Part model, mm, in its own coordinate system. A direction names the side the tool comes from. Round coordinates to 2 decimals unless told otherwise and drop trailing zeros. Write each loop counter-clockwise with the first axis right and the second up, starting at its lowest first coordinate (ties: lowest second). Pieces come first, ordered by that corner, then holes. Notation, with made-up numbers: M 37.5,69.5 L 81.5,69.5 A25 cw 81.5,91.5 Z; hole C 27.25,26 d8. An arc over 180 degrees is marked long. Use a Markdown table: item, result. Add a question column.
1) Which spindle directions (+Z, -Z, +X, -X, +Y, -Y) get a long thin tool onto all of the face, cutting with end or side? Do faces 5 (the face through (10, 31.1, -15)), 6 (the face through (22.1, 4.5, -13)), 7 (the face through (7.535, 129.651, -14.58)). Say none if no direction does.
2) Slice it at D-D on z = -15. Give the number of separate pieces and of enclosed holes in the cut face, plus the area to 3 significant figures.
3) Wall check: probe 1 along Y at (x, z) = (25, -15) (3 decimals); probe 2 along Y at (x, z) = (21.45, -15) (1 decimal); probe 3 along Z at (x, y) = (24, 23.56). Give the ranges that are in metal, low to high.
4) Two-plate mould, pull along Z, no slides. Class faces 1 (the face through (22.1, 21.5, -13)), 2 (the face through (15, 28, -30)), 3 (the face through (5.39, 116.48, -14.58)), 4 (the face through (15, 28, 0)): released by +Z, released by -Z, zero draft, split by the parting line, or undercut.
5) Slice it at A-A on y = 15.06. Write the cut outline in (x, z) (3 decimals).
6) Slice it at C-C on x = 26.5. Write the cut outline in (y, z) (3 decimals), plus the area to 3 significant figures.
7) Drop flat-ended pins along their axis: P1, Ø7.5, axis at y = 6.5, z = -12.5, coming from the -X side; P2, Ø3, axis at x = 26, y = -7.5, coming from the -Z side (3 decimals); P3, Ø4.5, axis at x = 16.5, z = -37.5, coming from the -Y side. Give the stop position or say it passes through.
8) Slice it at B-B on z = 10.5. Write the cut outline in (x, y), plus the area to 3 significant figures.
Autodesk Inventor part; units mm, degrees
ref_plane "Work Plane1" through (0, 0, -15) normal (0, 0, 1) x (1, 0, 0)
ref_plane "YZ Plane" through (0, 0, 0) normal (1, 0, 0) x (0, 1, 0)
ref_plane "XZ Plane" through (0, 0, 0) normal (0, 1, 0) x (-1, 0, 0)
sketch "Sketch1" plane through (0, 0, 0) normal (0, 0, 1) x (1, 0, 0)
  line L0 (0, 0) -> (25, 0)
  line L1 (25, 0) -> (25, 40)
  line L2 (25, 40) -> (0, 40)
  line L3 (0, 40) -> (0, 0)
  dimension "d1" = 25
  dimension "d2" = 40
  dimension "d3" = 25
extrude "Extrusion1" add sketch "Sketch1" against normal blind 30
sketch "Sketch2" plane through (25, 0, 0) normal (1, 0, 0) x (0, 0, -1)
  line L0 (0, 0) -> (30, 0)
  circle A0 centre (15, 6.56) radius 2.46
extrude "Extrusion2" cut sketch "Sketch2" against normal blind 30
sketch "Sketch3" plane through (0, 0, 0) normal (-1, 0, 0) x (0, 0, 1)
  line L0 (0, 0) -> (-30, 0)
  line L1 (-25.05, 0) -> (-4.95, 0)
  line L2 (-4.95, 0) -> (-4.95, 33.12)
  line L3 (-4.95, 33.12) -> (-25.05, 33.12)
  line L4 (-25.05, 33.12) -> (-25.05, 0)
  dimension "d11" = 20.1
extrude "Extrusion3" cut sketch "Sketch3" against normal blind 20
sketch "Sketch4" plane through (0, 0, 0) normal (0, -1, 0) x (1, 0, 0)
  line L0 (20, -4.95) -> (20, -25.05)
  line L1 (20, -15) -> (25, -15)
  line L2 (25, 0) -> (25, -30)
  line L3 (20, -8.025) -> (25, -8.025)
  line L4 (25, -8.025) -> (25, -21.975)
  line L5 (25, -21.975) -> (20, -21.975)
  line L6 (20, -21.975) -> (20, -8.025)
  line L7 (20, -8.025) -> (25, -21.975) construction
  line L8 (25, -8.025) -> (20, -21.975) construction
  line L9 (25, -12.54) -> (25, -17.46)
  point P0 (0, 0)
  point P1 (22.5, -15)
  dimension "d14" = 13.95
extrude "Extrusion4" add sketch "Sketch4" along normal blind 15
sketch "Sketch5" plane through (20, 0, 0) normal (-1, 0, 0) x (0, 0, 1)
  circle A0 centre (-15, 6.56) radius 2.46
  circle A1 centre (-15, 6.56) radius 4.7025
  circle A2 centre (-15, 6.56) radius 2.46
  circle A3 centre (-15, 6.56) radius 2.46
  point P0 (0, 0)
  dimension "d17" = 9.405
extrude "Extrusion5" cut sketch "Sketch5" against normal blind 2.1
sketch "Sketch6" plane through (25, 0, 0) normal (1, 0, 0) x (0, 0, -1)
  circle A0 centre (15, 6.56) radius 4.7025
  line L0 (15, 6.56) -> (15, 23.56)
  circle A1 centre (15, 23.56) radius 2.46
  point P0 (0, 0)
  dimension "d20" = 17
  dimension "d21" = 4.92
extrude "Extrusion6" cut sketch "Sketch6" against normal blind 10 contours A1
sketch "Sketch7" plane through (20, 0, 0) normal (-1, 0, 0) x (0, 0, 1)
  circle A0 centre (-15, 23.56) radius 2.46
  circle A1 centre (-15, 23.56) radius 4.7025
  point P0 (0, 0)
  dimension "d24" = 9.405
extrude "Extrusion7" cut sketch "Sketch7" against normal blind 2.1
sketch "Sketch9" plane through (25, 0, 0) normal (1, 0, 0) x (0, 0, -1)
  circle A0 centre (15, 6.56) radius 2.46
  circle A1 centre (15, 6.56) radius 2.46
  circle A2 centre (15, 23.56) radius 2.46
  circle A3 centre (15, 23.56) radius 2.46
  line L0 (30, 40) -> (30, 0)
  line L1 (30, 0) -> (30, 40)
  line L2 (30, 40) -> (0, 40)
  line L3 (0, 40) -> (0, 0)
  line L4 (0, 0) -> (8.025, 0)
  line L5 (21.975, 0) -> (21.975, -15)
  line L6 (21.975, -15) -> (8.025, -15)
  line L7 (8.025, -15) -> (8.025, 0)
  line L8 (0, 0) -> (8.025, 0)
  line L9 (21.975, 0) -> (30, 0)
extrude "Extrusion8" add sketch "Sketch9" along normal blind 5
sketch "Sketch10" plane through (0, 40, 0) normal (0, 1, 0) x (1, 0, 0)
  line L0 (0, 30) -> (30, 30)
  line L1 (30, 0) -> (0, 0)
  line L2 (0, 30) -> (30, 30)
  line L3 (30, 30) -> (30, 0)
  line L4 (30, 0) -> (0, 0)
  line L5 (0, 0) -> (0, 30)
extrude "Extrusion9" add sketch "Sketch10" along normal blind 30
sketch "Sketch12" plane through (30, 0, 0) normal (1, 0, 0) x (0, 0, -1)
  circle A0 centre (15, 6.56) radius 2.46
  line L0 (15, 6.56) -> (15, 15.06)
  circle A1 centre (15, 15.06) radius 2.525
  point P0 (0, 0)
  dimension "d31" = 8.5
  dimension "d33" = 5.05
extrude "Extrusion10" cut sketch "Sketch12" against normal blind 30 contours A1
sketch "Sketch15" plane through (0, 0, -25.05) normal (-1, 0, 0) x (0, 0, 1)
  line L0 (0, 33.12) -> (20.1, 33.12)
  line L1 (20.1, 33.12) -> (20.1, 0)
  line L2 (0, 33.12) -> (20.1, 33.12)
  line L3 (20.1, 33.12) -> (20.1, 31.1)
  line L4 (20.1, 31.1) -> (0, 31.1)
  line L5 (0, 31.1) -> (0, 33.12)
  point P0 (25.05, 0)
  dimension "d57" = 2.02
extrude "Extrusion13" add sketch "Sketch15" against normal blind 20
sketch "Sketch17" plane through (0, 0, 0) normal (0, 0, 1) x (1, 0, 0)
  line L0 (0, 70) -> (30, 70)
  line L1 (30, 70) -> (50.0622, 90.0622)
  line L2 (30, 70) -> (80, 70) construction
  line L3 (11.9522, 97.2454) -> (0, 85.2932)
  line L4 (0, 70) -> (0, 85.2932)
  line L5 (0, 70) -> (0, 0)
  line L6 (0, 70) -> (30, 70)
  line L7 (10.923, 112.2849) -> (0, 120.567)
  line L8 (50.0622, 105.3553) -> (50.0622, 120.567)
  line L9 (50.0622, 105.3553) -> (50.0622, 90.0622)
  arc A0 (11.9522, 97.2454) -> (10.923, 112.2849) centre (4.8811, 104.3165) ccw
  line L10 (0, 150.567) -> (30, 150.567)
  line L11 (30, 150.567) -> (50.0622, 120.567)
  line L12 (5, 147.567) -> (0, 150.567)
  line L13 (5, 123.567) -> (0, 120.567)
  line L14 (5, 123.567) -> (10, 135.567)
  line L15 (10, 135.567) -> (5, 147.567)
  dimension "d61" = 45
  dimension "d62" = 32.0271
  dimension "d72" = 10
extrude "Extrusion14" add sketch "Sketch17" against normal blind 30
sketch "Sketch22" plane through (0, 0, 0) normal (0, 0, 1) x (1, 0, 0)
  line L0 (30, 0) -> (30, 70)
  line L1 (50.0622, 120.567) -> (50.0622, 90.0622)
  line L2 (30, 70) -> (50.0622, 90.0622)
  line L3 (50.0622, 90.0622) -> (50.0622, 120.567)
  line L4 (50.0622, 120.567) -> (30, 150.567)
  line L5 (50.0622, 120.567) -> (30, 150.567)
  line L6 (30, 150.567) -> (0, 150.567)
  line L7 (30, 150.567) -> (0, 150.567)
  line L8 (0, 150.567) -> (5, 147.567)
  line L9 (0, 150.567) -> (5, 147.567)
  line L10 (5, 147.567) -> (10, 135.567)
  line L11 (5, 147.567) -> (10, 135.567)
  line L12 (5, 123.567) -> (10, 135.567)
  line L13 (10, 135.567) -> (5, 123.567)
  line L14 (5, 123.567) -> (0, 120.567)
  line L15 (5, 123.567) -> (0, 120.567)
  line L16 (10.923, 112.2849) -> (0, 120.567)
  line L17 (0, 120.567) -> (10.923, 112.2849)
  line L18 (0, 85.2932) -> (11.9522, 97.2454)
  line L19 (11.9522, 97.2454) -> (0, 85.2932)
  line L20 (0, 85.2932) -> (0, 55.2932)
  line L21 (0, 0) -> (0, 85.2932)
  line L22 (0, 55.2932) -> (30, 55.2932)
  line L23 (30, 55.2932) -> (30, 70)
  arc A0 (11.9522, 97.2454) -> (10.923, 112.2849) centre (4.8811, 104.3165) ccw
  arc A1 (11.9522, 97.2454) -> (10.923, 112.2849) centre (4.8811, 104.3165) ccw
  dimension "d87" = 30
extrude "Extrusion15" add sketch "Sketch22" along normal blind 15
ref_plane "Work Plane1" through (0, 0, -15) normal (0, 0, 1) x (1, 0, 0)
mirror "Mirror1" about plane through (0, 0, -15) normal (0, 0, 1) of "Extrusion15"
properties part number "rec_c_24mm_x_60mm"
Entries:
| question | item | result |
|---|---|---|
| 1 | face 5 | -X, -Y |
| 1 | face 6 | -X |
| 1 | face 7 | +Z, -Z, -X |
| 2 | separate pieces | 4 |
| 2 | enclosed holes | 0 |
| 2 | area | 4,470 mm^2 |
| 3 | probe 1 | y = -15 to 4.1, 9.02 to 12.535, 17.585 to 21.1, 26.02 to 150.567 |
| 3 | probe 2 | y = -15 to 1.9, 11.3 to 12.5, 17.6 to 18.9, 28.3 to 150.6 |
| 3 | probe 3 | z = -30 to -17.46, -12.54 to 0 |
| 4 | face 1 | undercut |
| 4 | face 2 | released by -Z |
| 4 | face 3 | zero draft |
| 4 | face 4 | released by +Z |
| 5 | outline | M 0,-30 L 30,-30 L 30,-17.525 L 20,-17.525 L 20,-25.05 L 0,-25.05 Z; M 0,-4.95 L 20,-4.95 L 20,-12.475 L 30,-12.475 L 30,0 L 0,0 Z |
| 6 | outline | M -15,-21.975 L 0,-21.975 L 0,-30 L 55.293,-30 L 55.293,-45 L 150.567,-45 L 150.567,15 L 55.293,15 L 55.293,0 L 0,0 L 0,-8.025 L -15,-8.025 Z; hole C 6.56,-15 d4.92; hole C 15.06,-15 d5.05; hole C 23.56,-15 d4.92 |
| 6 | area | 7,530 mm^2 |
| 7 | P1 | stops at x = 20 |
| 7 | P2 | stops at z = -21.975 |
| 7 | P3 | stops at y = 55.29 |
| 8 | outline | M 0,55.29 L 30,55.29 L 30,70 L 50.06,90.06 L 50.06,120.57 L 30,150.57 L 0,150.57 L 5,147.57 L 10,135.57 L 5,123.57 L 0,120.57 L 10.92,112.28 A10 cw 11.95,97.25 L 0,85.29 Z |
| 8 | area | 3,450 mm^2 |
